Geometry check sheet. Reference: the model listing, model coordinates, mm. Face numbers are marked on the shaded views. A direction names the side the tool comes from. Give positions to 0.01 mm unless a question says otherwise; leave off trailing zeros. Write each loop counter-clockwise with the first axis right and the second up, starting at its lowest first coordinate (ties: lowest second). Pieces come first, ordered by that corner, then holes. Notation, with made-up numbers: (-18.5, 85.25) -> (25.5, 85.25) arc R24 ccw to (25.5, 114.25) -> close; hole circle Ø9 at (72.5, 63). An arc over 180 degrees is marked (long way). Use a Markdown table: item, result. Add a question column.
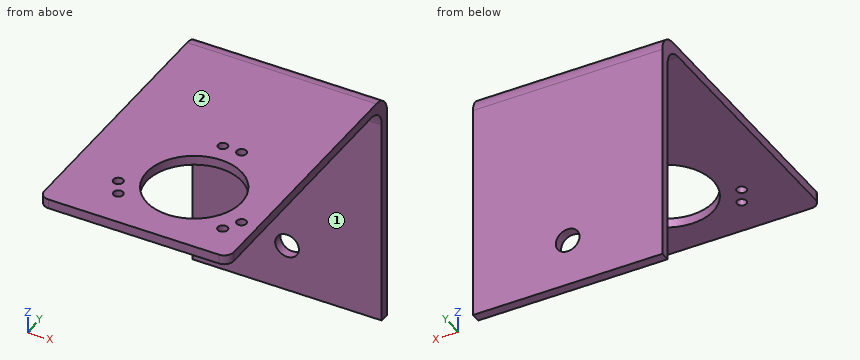
from build123d import *

# Parameters (mm, degrees)
SKETCH1_W           = 40
SKETCH1_H           = 42
BOSS_EXTRUDE1_DEPTH = 2
SKETCH3_W           = 40
SKETCH3_H           = 2
BOSS_EXTRUDE2_DEPTH = 48.3
FILLET1_R           = 2
FILLET2_R           = 2
CUT_EXTRUDE5_REACH  = 52.3
SKETCH7_R           = 1.008522139
SKETCH7_R_2         = 1.026344308
SKETCH7_R_3         = 1.008522138
SKETCH7_R_4         = 10
CUT_EXTRUDE6_REACH  = 4
SKETCH4_R           = 2.5
SKETCH8_W           = 40
SKETCH8_H           = 50.3
SKETCH8_R           = 2.5
BOSS_EXTRUDE3_DEPTH = 18.05
SKETCH10_W          = 40
SKETCH10_H          = 6.748630519
BOSS_EXTRUDE5_DEPTH = 17.05
SKETCH11_W          = 40
SKETCH11_H          = 46.3
CUT_EXTRUDE7_DEPTH  = 18.05
SKETCH12_W          = 40
SKETCH12_H          = 2
CUT_EXTRUDE8_DEPTH  = 22.05
SKETCH13_W          = 2
SKETCH13_H          = 2
BOSS_EXTRUDE6_DEPTH = 40
FILLET3_R           = 4
FILLET4_R           = 4


with BuildPart() as part:
    # Sketch1 → Boss-Extrude1 (new body)
    with BuildSketch(Plane.XY):
        Rectangle(SKETCH1_W, SKETCH1_H)
    extrude(amount=BOSS_EXTRUDE1_DEPTH)

    # Sketch3 → Boss-Extrude2 (add)
    with BuildSketch(Plane(origin=(0, 0, 0), x_dir=(-1, 0, 0), z_dir=(0, 0, -1))):
        with Locations((0, 20)):
            Rectangle(SKETCH3_W, SKETCH3_H)
    extrude(amount=BOSS_EXTRUDE2_DEPTH)

    # Fillet1
    fillet1_edges = [part.edges().sort_by_distance(p)[0] for p in [
        (0, 19, 0),
        (0, 21, 2),
    ]]
    fillet(fillet1_edges, radius=FILLET1_R)

    # Fillet2
    fillet2_edges = [part.edges().sort_by_distance(p)[0] for p in [
        (20, -21, 1),
        (-20, -21, 1),
    ]]
    fillet(fillet2_edges, radius=FILLET2_R)

    # Sketch7 → Cut-Extrude5 (cut, up to next)
    with BuildSketch(Plane.XY.offset(2), mode=Mode.PRIVATE) as cut_extrude5_sk1:
        with Locations((-7.700271416, -13.062366093)):
            Circle(SKETCH7_R)
    cut_extrude5_tool1 = extrude(cut_extrude5_sk1.sketch, amount=-CUT_EXTRUDE5_REACH, mode=Mode.PRIVATE) & part.part
    add(cut_extrude5_tool1.solids().sort_by_distance((-7.700271, -13.062366, 2))[0], mode=Mode.SUBTRACT)
    # Sketch7 → Cut-Extrude5 (cut, up to next)
    with BuildSketch(Plane.XY.offset(2), mode=Mode.PRIVATE) as cut_extrude5_sk2:
        with Locations((-9.646314877, -9.567667988)):
            Circle(SKETCH7_R_2)
    cut_extrude5_tool2 = extrude(cut_extrude5_sk2.sketch, amount=-CUT_EXTRUDE5_REACH, mode=Mode.PRIVATE) & part.part
    add(cut_extrude5_tool2.solids().sort_by_distance((-9.646315, -9.567668, 2))[0], mode=Mode.SUBTRACT)
    # Sketch7 → Cut-Extrude5 (cut, up to next)
    with BuildSketch(Plane.XY.offset(2), mode=Mode.PRIVATE) as cut_extrude5_sk3:
        with Locations((1.782545423, 9.537272948)):
            Circle(SKETCH7_R_3)
    cut_extrude5_tool3 = extrude(cut_extrude5_sk3.sketch, amount=-CUT_EXTRUDE5_REACH, mode=Mode.PRIVATE) & part.part
    add(cut_extrude5_tool3.solids().sort_by_distance((1.782545, 9.537273, 2))[0], mode=Mode.SUBTRACT)
    # Sketch7 → Cut-Extrude5 (cut, up to next)
    with BuildSketch(Plane.XY.offset(2), mode=Mode.PRIVATE) as cut_extrude5_sk4:
        with Locations((5.782064491, 9.475246969)):
            Circle(SKETCH7_R_2)
    cut_extrude5_tool4 = extrude(cut_extrude5_sk4.sketch, amount=-CUT_EXTRUDE5_REACH, mode=Mode.PRIVATE) & part.part
    add(cut_extrude5_tool4.solids().sort_by_distance((5.782064, 9.475247, 2))[0], mode=Mode.SUBTRACT)
    # Sketch7 → Cut-Extrude5 (cut, up to next)
    with BuildSketch(Plane.XY.offset(2), mode=Mode.PRIVATE) as cut_extrude5_sk5:
        with Locations((3.565090845, -4.5)):
            Circle(SKETCH7_R_4)
    cut_extrude5_tool5 = extrude(cut_extrude5_sk5.sketch, amount=-CUT_EXTRUDE5_REACH, mode=Mode.PRIVATE) & part.part
    add(cut_extrude5_tool5.solids().sort_by_distance((3.565091, -4.5, 2))[0], mode=Mode.SUBTRACT)
    # Sketch7 → Cut-Extrude5 (cut, up to next)
    with BuildSketch(Plane.XY.offset(2), mode=Mode.PRIVATE) as cut_extrude5_sk6:
        with Locations((16.612998529, -9.974906855)):
            Circle(SKETCH7_R)
    cut_extrude5_tool6 = extrude(cut_extrude5_sk6.sketch, amount=-CUT_EXTRUDE5_REACH, mode=Mode.PRIVATE) & part.part
    add(cut_extrude5_tool6.solids().sort_by_distance((16.612999, -9.974907, 2))[0], mode=Mode.SUBTRACT)
    # Sketch7 → Cut-Extrude5 (cut, up to next)
    with BuildSketch(Plane.XY.offset(2), mode=Mode.PRIVATE) as cut_extrude5_sk7:
        with Locations((14.559522922, -13.407578981)):
            Circle(SKETCH7_R_2)
    cut_extrude5_tool7 = extrude(cut_extrude5_sk7.sketch, amount=-CUT_EXTRUDE5_REACH, mode=Mode.PRIVATE) & part.part
    add(cut_extrude5_tool7.solids().sort_by_distance((14.559523, -13.407579, 2))[0], mode=Mode.SUBTRACT)

    # Sketch4 → Cut-Extrude6 (cut, up to next)
    with BuildSketch(Plane.XZ.offset(-19), mode=Mode.PRIVATE) as cut_extrude6_sk1:
        with Locations((0, -38.3)):
            Circle(SKETCH4_R)
    cut_extrude6_tool1 = extrude(cut_extrude6_sk1.sketch, amount=-CUT_EXTRUDE6_REACH, mode=Mode.PRIVATE) & part.part
    add(cut_extrude6_tool1.solids().sort_by_distance((0, 19, -38.3))[0], mode=Mode.SUBTRACT)

    # Sketch8 → Boss-Extrude3 (add)
    with BuildSketch(Plane(origin=(0, 21, 0), x_dir=(1, 0, 0), z_dir=(0, 1, 0))):
        with Locations((0, 23.15)):
            Rectangle(SKETCH8_W, SKETCH8_H)
        with Locations((0, 38.3)):
            Circle(SKETCH8_R, mode=Mode.SUBTRACT)
    extrude(amount=BOSS_EXTRUDE3_DEPTH)

    # Sketch10 → Boss-Extrude5 (add)
    with BuildSketch(Plane.XY.offset(2)):
        with Locations((0, 22.37431526)):
            Rectangle(SKETCH10_W, SKETCH10_H)
    extrude(amount=-BOSS_EXTRUDE5_DEPTH)

    # Sketch11 → Cut-Extrude7 (cut)
    with BuildSketch(Plane.XZ.offset(-19)):
        with Locations((0, -25.15)):
            Rectangle(SKETCH11_W, SKETCH11_H)
    extrude(amount=-CUT_EXTRUDE7_DEPTH, mode=Mode.SUBTRACT)

    # Sketch12 → Cut-Extrude8 (cut)
    with BuildSketch(Plane(origin=(0, 39.05, 0), x_dir=(1, 0, 0), z_dir=(0, 1, 0))):
        with Locations((0, 1)):
            Rectangle(SKETCH12_W, SKETCH12_H)
    extrude(amount=-CUT_EXTRUDE8_DEPTH, mode=Mode.SUBTRACT)

    # Sketch13 → Boss-Extrude6 (add)
    with BuildSketch(Plane(origin=(20, 0, 0), x_dir=(0, 0, -1), z_dir=(1, 0, 0))):
        with Locations((1, 38.05)):
            Rectangle(SKETCH13_W, SKETCH13_H)
    extrude(amount=-BOSS_EXTRUDE6_DEPTH)

    # Fillet3
    fillet3_edges = [part.edges().sort_by_distance(p)[0] for p in [
        (0, 39.05, 2),
    ]]
    fillet(fillet3_edges, radius=FILLET3_R)

    # Fillet4
    fillet4_edges = [part.edges().sort_by_distance(p)[0] for p in [
        (0, 37.05, 0),
    ]]
    fillet(fillet4_edges, radius=FILLET4_R)


solid = part.part
1) Sectioned sample at A-A, the plane z = -38.3. Enter the section's corners in (x, y).
2) Sectioned sample at D-D, the plane x = -13.5. Enter the section's corners in (y, z).
3) Material ranges on probe 1 along X at (y, z) = (38, -38); probe 2 along Z at (x, y) = (-5.5, 31); probe 3 along Y at (x, z) = (-17.5, -14.5), recorded low to high. Write a range as [from, to].
4) Gauge pin test, flat ends, axial feed: P1, Ø2.5, axis at x = -7.7, y = -13.06, coming from the -Z side; P2, Ø5, axis at x = 13.5, z = -32, coming from the -Y side; P3, Ø6, axis at x = 0, z = -38.3, coming from the +Y side; P4, Ø1.8, axis at x = 1.78, y = 9.54, coming from the -Z side. Record the tip position at first contact, or that the pin passes through.
5) Tool access check on the marked faces 1 and 2. Record the directions out of +Z, -Z, +X, -X, +Y, -Y that give a thin tool (end or side, any length) a straight path to the whole face; none if there is none.
6) Sectioned sample at B-B, the plane y = -4.5. Enter the section's corners in (x, z).
7) Sectioned sample at C-C, the plane x = 0. Enter the section's corners in (y, z), and give its area (3 significant figures).
Check values:
| question | item | result |
|---|---|---|
| 1 | outline | (-20, 37.05) -> (-2.5, 37.05) -> (-2.5, 39.05) -> (-20, 39.05) -> close; (2.5, 37.05) -> (20, 37.05) -> (20, 39.05) -> (2.5, 39.05) -> close |
| 2 | outline | (-21, 0) -> (33.05, 0) arc R4 cw to (37.05, -4) -> (37.05, -48.3) -> (39.05, -48.3) -> (39.05, -2) arc R4 ccw to (35.05, 2) -> (-21, 2) -> close |
| 3 | probe 1 | [-20, -2.48], [2.48, 20] |
| 3 | probe 2 | [0, 2] |
| 3 | probe 3 | [37.05, 39.05] |
| 4 | P1 | z = 0 |
| 4 | P2 | y = 37.05 |
| 4 | P3 | y = 39.05 |
| 4 | P4 | through |
| 5 | face 1 | -Z, +X, -X, -Y |
| 5 | face 2 | +Z, +X, -X, +Y, -Y |
| 6 | outline | (-20, 0) -> (-6.43, 0) -> (-6.43, 2) -> (-20, 2) -> close; (13.57, 0) -> (20, 0) -> (20, 2) -> (13.57, 2) -> close |
| 7 | outline | (-21, 0) -> (-13.84, 0) -> (-13.84, 2) -> (-21, 2) -> close; (4.84, 0) -> (33.05, 0) arc R4 cw to (37.05, -4) -> (37.05, -35.8) -> (39.05, -35.8) -> (39.05, -2) arc R4 ccw to (35.05, 2) -> (4.84, 2) -> close; (37.05, -48.3) -> (39.05, -48.3) -> (39.05, -40.8) -> (37.05, -40.8) -> close |
| 7 | area | 169 mm² |
